Build history of the part. All positions in model axes, mm. Give positions to 0.01 mm unless a question says otherwise; leave off trailing zeros. Order: outer loops, then holes, each group sorted by start corner. A loop starts at its lowest first (then second) coordinate and runs counter-clockwise, first axis right, second up. Notation, with made-up numbers: (-15.5, 45) -> (20.5, 45) arc R12 cw to (20.5, 55) -> close; hole circle Ø11 at (55, 67.5). An arc over 180 degrees is marked (long way). Use a Markdown table: item, result. Add a question column.
```python
from build123d import *

# Parameters (mm, degrees)
BOSS_EXTRUDE1_DEPTH     = 514.48335
SKETCH2_R               = 3.175
CUT_EXTRUDE1_DEPTH      = 1
CUT_EXTRUDE1_DEPTH_BACK = 515.48335
SKETCH3_R               = 3.175
BOSS_EXTRUDE2_DEPTH     = 571.5


with BuildPart() as part:
    # Sketch1 → Boss-Extrude1 (new body)
    with BuildSketch(Plane.XY):
        Polygon((-7.332348419, 0), (-3.666174209, -6.35), (3.666174209, -6.35), (7.332348419, 0), (3.666174209, 6.35), (-3.666174209, 6.35), align=None)
    extrude(amount=BOSS_EXTRUDE1_DEPTH)

    # Sketch2 → Cut-Extrude1 (cut, two sides)
    with BuildSketch(Plane.XY.offset(514.48335)) as cut_extrude1_sk:
        Circle(SKETCH2_R)
    extrude(amount=CUT_EXTRUDE1_DEPTH, mode=Mode.SUBTRACT)
    extrude(cut_extrude1_sk.sketch, amount=-CUT_EXTRUDE1_DEPTH_BACK, mode=Mode.SUBTRACT)

    # Sketch3 → Boss-Extrude2 (add)
    with BuildSketch(Plane.XY.offset(514.48335)):
        Polygon((-3.666174209, -6.35), (3.666174209, -6.35), (7.332348419, 0), (3.666174209, 6.35), (-3.666174209, 6.35), (-7.332348419, 0), align=None)
        Circle(SKETCH3_R, mode=Mode.SUBTRACT)
    extrude(amount=-BOSS_EXTRUDE2_DEPTH)


solid = part.part
```
(1) Wall check: probe 1 along Y at (x, z) = (0, 139) (3 decimals); probe 2 along Y at (x, z) = (-0.5, 180); probe 3 along X at (y, z) = (-2.75, 77). Give the ranges that are in metal, low to high.
(2) Band-saw the part on B-B on x = 0. Give the cut face in (y, z) (3 decimals).
(3) Band-saw the part on A-A on z = 143.5. Give the cut face in (x, y) (3 decimals).
(4) Pin check, flat tips, straight feed: pin 1 Ø3 at (y, z) = (-4.5, 127.5) entering from -X; pin 2 Ø5 at (y, z) = (2, 228) entering from +X; pin 3 Ø5 at (x, y) = (0, 0) entering from +Z; pin 4 Ø1 at (x, z) = (-5.5, 289) entering from -Y. Stop position of each tip, or through.
Response:
| question | item | result |
|---|---|---|
| 1 | probe 1 | y = -6.35 to -3.175, 3.175 to 6.35 |
| 1 | probe 2 | y = -6.35 to -3.14, 3.14 to 6.35 |
| 1 | probe 3 | x = -5.74 to -1.59, 1.59 to 5.74 |
| 2 | outline | (-6.35, -57.017) -> (-3.175, -57.017) -> (-3.175, 514.483) -> (-6.35, 514.483) -> close; (3.175, -57.017) -> (6.35, -57.017) -> (6.35, 514.483) -> (3.175, 514.483) -> close |
| 3 | outline | (-7.332, 0) -> (-3.666, -6.35) -> (3.666, -6.35) -> (7.332, 0) -> (3.666, 6.35) -> (-3.666, 6.35) -> close; hole circle Ø6.35 at (0, 0) |
| 4 | pin 1 | stops at x = -5.6 |
| 4 | pin 2 | stops at x = 7.33 |
| 4 | pin 3 | passes through |
| 4 | pin 4 | stops at y = -4.04 |
